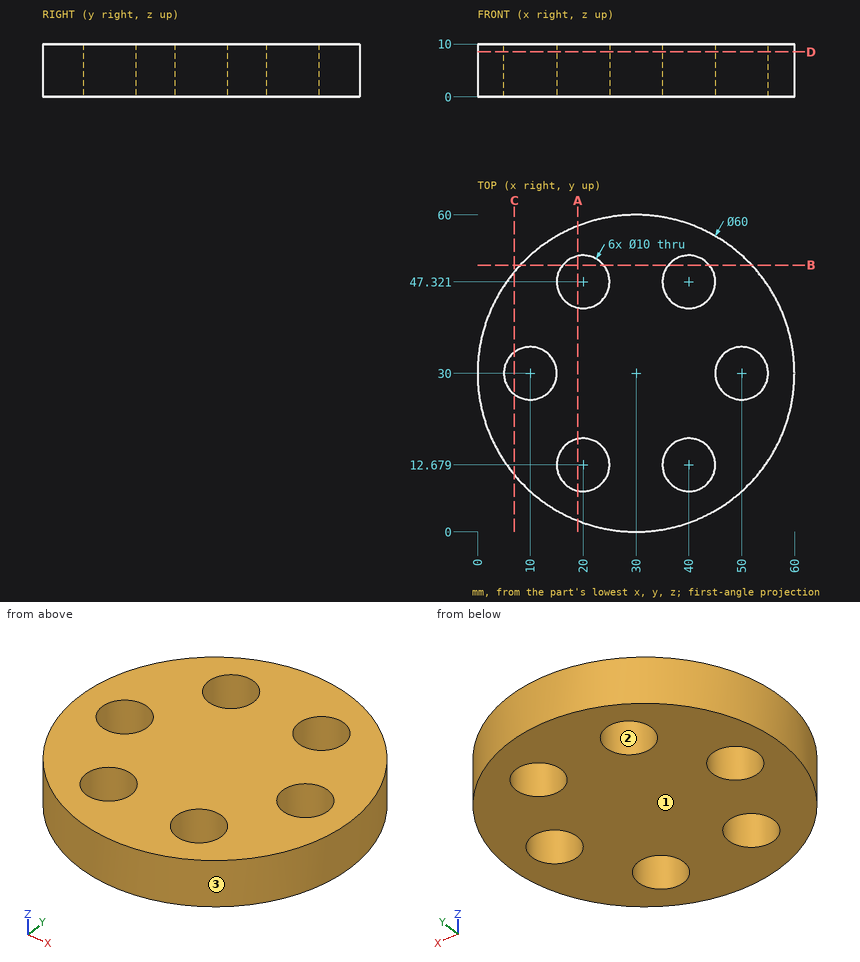
Input: dimensioned drawing with shaded views. Units: mm. Origin: part minimum x, y, z. Coordinates: 2 decimals unless noted, no trailing zeros. Loops run counter-clockwise (first coordinate to the right, second up) from the corner with the lowest first, then second, coordinate; pieces in that order, holes last. Notation, with made-up numbers: M -27.5,23 L -10.5,23 A11 ccw -10.5,27 Z; hole C 85.5,7 d11. An arc over 180 degrees is marked long. One line per item, written item: value. Start each with the question number.
1) Material intervals for L1, parallel to Y at x = 40, z = 7 (1 decimal); L2, parallel to X at y = 31.5, z = 6; L3, parallel to X at y = 28, z = 7 (1 decimal), sorted ascending. Write a range as from..to.
2) Cut plane D-D (z = 8.5). Return loops of the section in (x, y).
3) Cut plane A-A (x = 19). Return loops of the section in (y, z), then the cut area to 3 significant figures.
4) Cut plane B-B (y = 50.5). Return loops of the section in (x, z).
5) Cut plane C-C (x = 7). Return loops of the section in (y, z), then the cut area to 3 significant figures.
6) Draft query along X for the marked faces 1, 2 and 3. Return one class per face: released by +X, released by -X, zero draft, split by the parting line, or undercut.
7) Pin query (flat end, axial travel): P1, Ø1.5, axis at x = 46, y = 26, coming from the -Z side; P2, Ø3, axis at x = 48.5, z = 4.5, coming from the -Y side; P3, Ø1.5, axis at y = 44.5, z = 2, coming from the +X side; P4, Ø4, axis at y = 11.5, z = 4.5, coming from the +X side (1 decimal). Return the tip coordinate at first contact, or that it passes through.
Evaluation:
1. L1: 1.7..7.7, 17.7..42.3, 52.3..58.3
1. L2: 0.04..5.23, 14.77..45.23, 54.77..59.96
1. L3: 0.1..5.4, 14.6..45.4, 54.6..59.9
2. outline: C 30,30 d60; hole C 10,30 d10; hole C 20,12.68 d10; hole C 20,47.32 d10; hole C 40,12.68 d10; hole C 40,47.32 d10; hole C 50,30 d10
3. outline: M 2.09,0 L 7.78,0 L 7.78,10 L 2.09,10 Z; M 17.58,0 L 42.42,0 L 42.42,10 L 17.58,10 Z; M 52.22,0 L 57.91,0 L 57.91,10 L 52.22,10 Z
3. area: 362 mm^2
4. outline: M 8.1,0 L 16.14,0 L 16.14,10 L 8.1,10 Z; M 23.86,0 L 36.14,0 L 36.14,10 L 23.86,10 Z; M 43.86,0 L 51.9,0 L 51.9,10 L 43.86,10 Z
5. outline: M 10.74,0 L 26,0 L 26,10 L 10.74,10 Z; M 34,0 L 49.26,0 L 49.26,10 L 34,10 Z
5. area: 305 mm^2
6. face 1: zero draft
6. face 2: undercut
6. face 3: split by the parting line
7. P1: z = 0
7. P2: y = 5.28
7. P3: x = 56.66
7. P4: x = 55.1
